Build history of the part. All positions in model axes, mm. A direction names the side the tool comes from. Round coordinates to 2 decimals unless told otherwise and drop trailing zeros. Loops run counter-clockwise (first coordinate to the right, second up) from the corner with the lowest first, then second, coordinate; pieces in that order, holes last. Notation, with made-up numbers: M 89.5,79 L 146.5,79 A18 ccw 146.5,89 Z; hole C -5.75,-30 d3. An arc over 180 degrees is marked long. Use one line per item in the form item = value. Start each with the question number.
```python
from build123d import *

# Parameters (mm, degrees)
SKETCH6_W           = 24
SKETCH6_H           = 30
BOSS_EXTRUDE5_DEPTH = 35
CUT_EXTRUDE1_DEPTH  = 14.325
FILLET1_R           = 20
SKETCH11_R          = 1.65
CUT_EXTRUDE3_DEPTH  = 41.095199214
CUT_EXTRUDE8_DEPTH  = 14
SKETCH14_W          = 24
SKETCH14_H          = 50
BOSS_EXTRUDE6_DEPTH = 3.5
SKETCH15_R          = 2.1
CUT_EXTRUDE9_DEPTH  = 3.5
FILLET2_R           = 3


with BuildPart() as part:
    # Sketch6 → Boss-Extrude5 (new body)
    with BuildSketch(Plane(origin=(0, 0, 0), x_dir=(1, 0, 0), z_dir=(0, 1, 0))):
        Rectangle(SKETCH6_W, SKETCH6_H)
    extrude(amount=BOSS_EXTRUDE5_DEPTH)

    # Sketch8 → Cut-Extrude1 (cut)
    with BuildSketch(Plane(origin=(0, 17.5, 0), x_dir=(1, 0, 0), z_dir=(0, 1, 0))):
        Polygon((-12, 11.5), (-12, -15), (14.5, -15), align=None)
    cut_extrude1 = extrude(amount=-CUT_EXTRUDE1_DEPTH, mode=Mode.SUBTRACT)

    # Mirror2: Cut-Extrude1 across plane
    add(cut_extrude1.mirror(Plane.ZX.offset(17.5)), mode=Mode.SUBTRACT)

    # Fillet1
    fillet1_edges = [part.edges().sort_by_distance(p)[0] for p in [
        (-12, 1.5875, 15),
        (-12, 33.4125, 15),
    ]]
    fillet(fillet1_edges, radius=FILLET1_R)

    # Sketch11 → Cut-Extrude3 (cut, through all)
    with BuildSketch(Plane(origin=(-0.25, 0, 0.25), x_dir=(0.7071067811865439, 0, 0.7071067811865511), z_dir=(-0.7071067811865511, 0, 0.7071067811865439))):
        with Locations((4.084116139, 6.65)):
            Circle(SKETCH11_R)
        with Locations((4.084116139, 28.35)):
            Circle(SKETCH11_R)
    extrude(amount=-CUT_EXTRUDE3_DEPTH, mode=Mode.SUBTRACT)

    # Sketch12 → Cut-Extrude8 (cut)
    with BuildSketch(Plane(origin=(13.892135624, 0, -13.892135624), x_dir=(0.7071067811865439, 0, 0.7071067811865511), z_dir=(-0.7071067811865511, 0, 0.7071067811865439))):
        Polygon((6.784116139, 8.208845727), (4.084116139, 9.767691454), (1.384116139, 8.208845727), (1.384116139, 5.091154273), (4.084116139, 3.532308546), (6.784116139, 5.091154273), align=None)
        Polygon((6.784116139, 29.908845727), (6.784116139, 26.791154273), (4.084116139, 25.232308546), (1.384116139, 26.791154273), (1.384116139, 29.908845727), (4.084116139, 31.467691454), align=None)
    extrude(amount=CUT_EXTRUDE8_DEPTH, mode=Mode.SUBTRACT)

    # Sketch14 → Boss-Extrude6 (add)
    with BuildSketch(Plane(origin=(0, 0, -15), x_dir=(-1, 0, 0), z_dir=(0, 0, -1))):
        with Locations((0, 17.5)):
            Rectangle(SKETCH14_W, SKETCH14_H)
    extrude(amount=-BOSS_EXTRUDE6_DEPTH)

    # Sketch15 → Cut-Extrude9 (cut)
    with BuildSketch(Plane.XY.offset(-11.5)):
        with Locations((6, 38.75)):
            Circle(SKETCH15_R)
        with Locations((-6, 38.75)):
            Circle(SKETCH15_R)
        with Locations((-6, -3.75)):
            Circle(SKETCH15_R)
        with Locations((6, -3.75)):
            Circle(SKETCH15_R)
    extrude(amount=-CUT_EXTRUDE9_DEPTH, mode=Mode.SUBTRACT)

    # Fillet2
    fillet2_edges = [part.edges().sort_by_distance(p)[0] for p in [
        (12, -7.5, -13.25),
        (-12, 42.5, -13.25),
        (-12, -7.5, -13.25),
        (12, 42.5, -13.25),
    ]]
    fillet(fillet2_edges, radius=FILLET2_R)


solid = part.part
```
Q1. Saw through at C-C (x = 10). Give the cut face in (y, z) (3 decimals), and give its area (3 significant figures).
Q2. Saw through at B-B (x = -7). Give the cut face in (y, z) (3 decimals), and give its area (3 significant figures).
Q3. Saw through at A-A (y = -3.75). Give the cut face in (x, z), and give its area (3 significant figures).
Q4. Pull direction X, two halves, no side cores. Call faces 1 (the face through (0, -7.5, -13)), 2 (the face through (-11.1, -6.64, -13.23)), 3 (the face through (6.005, 5.308, -1.98)), 4 (the face through (8.535, 6.672, -6.577)): pulls with the +X half, pulls with the -X half, needs draft (parallel to the pull), parting line crosses it, or undercut.
Q5. Wall check: probe 1 along Y at (x, z) = (6, -12.7); probe 2 along Y at (x, z) = (-6, 1.5) (3 decimals); probe 3 along Y at (x, z) = (10, 9). Give the ranges that are in metal, low to high.
Q6. Drop flat-ended pins along their axis: P1, Ø6.5, axis at x = -6, y = 38.75, coming from the +Z side; P2, Ø7, axis at x = -3, z = 0, coming from the +Y side; P3, Ø7, axis at x = 0, z = 0.5, coming from the -Y side. Give the stop position or say it passes through.
Q7. Tool access for faces 5 (the face through (0, -4, -11.5)), 6 (the face through (8.7, 26, -4.8)), 7 (the face through (0, 35, 2)): list every direction of +Z, -Z, +X, -X, +Y, -Y with a clear straight run to the whole face (end or side of a thin tool).
Q8. Saw through at D-D (y = 17). Give the cut face in (x, z).
Filled in:
q1.outline = M -7.328,-15 L 42.328,-15 L 42.328,-11.5 L 35,-11.5 L 35,15 L 31.825,15 L 31.825,10.5 L 3.175,10.5 L 3.175,15 L 0,15 L 0,-11.5 L -7.328,-11.5 Z; hole M 3.532,-4.224 L 5.091,-8.043 L 8.209,-8.043 L 9.768,-4.224 L 8.209,-0.406 L 5.091,-0.406 Z; hole M 25.232,-4.224 L 26.791,-8.043 L 29.909,-8.043 L 31.468,-4.224 L 29.909,-0.406 L 26.791,-0.406 Z
q1.area = 901 mm²
q2.outline = M -7.5,-15 L -5.597,-15 L -5.597,-11.5 L -7.5,-11.5 Z; M -1.903,-15 L 36.903,-15 L 36.903,-11.5 L 35,-11.5 L 35,8.229 L 31.825,8.229 L 31.825,-6.5 L 3.175,-6.5 L 3.175,8.229 L 0,8.229 L 0,-11.5 L -1.903,-11.5 Z; M 40.597,-15 L 42.5,-15 L 42.5,-11.5 L 40.597,-11.5 Z
q2.area = 418 mm²
q3.outline = M -12,-15 L -8.1,-15 L -8.1,-11.5 L -12,-11.5 Z; M -3.9,-15 L 3.9,-15 L 3.9,-11.5 L -3.9,-11.5 Z; M 8.1,-15 L 12,-15 L 12,-11.5 L 8.1,-11.5 Z
q3.area = 54.6 mm²
q4.face_1 = needs draft
q4.face_2 = pulls with the -X half
q4.face_3 = undercut
q4.face_4 = pulls with the +X half
q5.probe_1 = -7.5 to -5.85, -1.65 to 36.65, 40.85 to 42.5
q5.probe_2 = 0 to 3.175, 31.825 to 35
q5.probe_3 = 0 to 35
q6.P1 = -11.5
q6.P2 = 35
q6.P3 = 0
q7.face_5 = +Z, +X, -X, -Y
q7.face_6 = none
q7.face_7 = +Z, +X, -X, +Y
q8.outline = M -12,-15 L 12,-15 L 12,12.5 L -12,-11.5 Z
